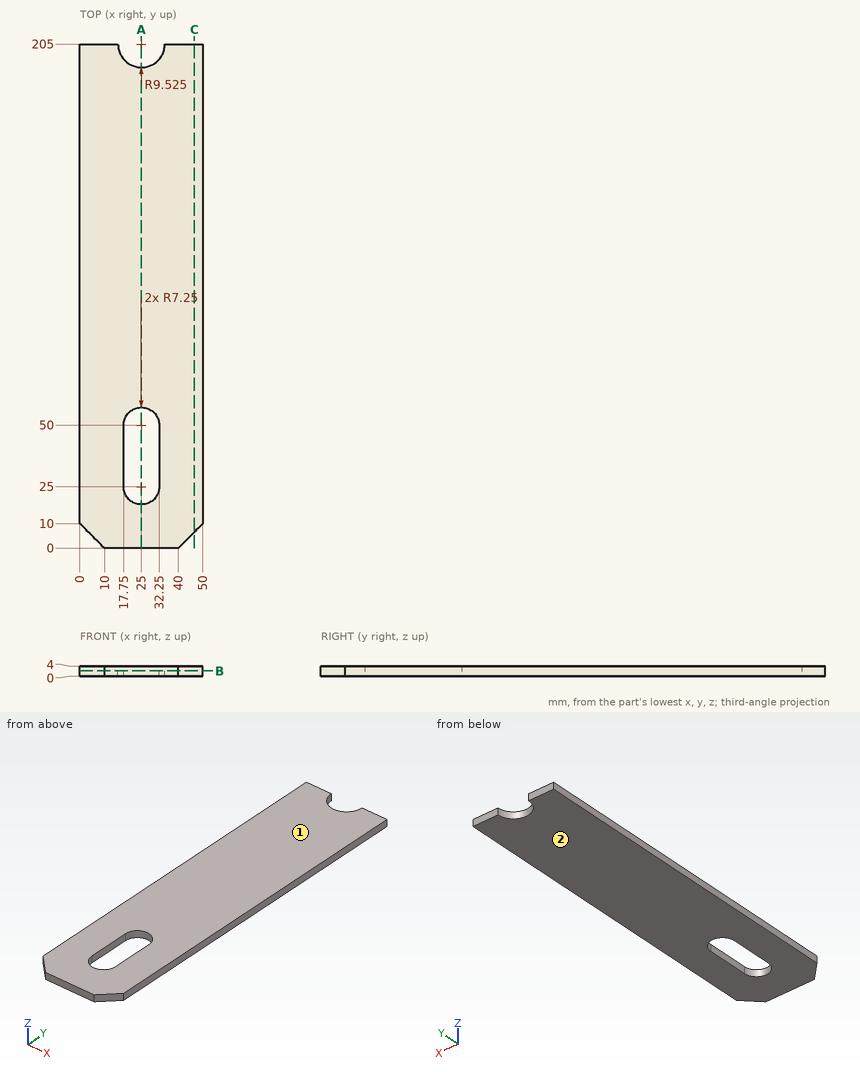
Verification items for this drawing (mm, ordinates from the low corner). Give positions to 0.01 mm unless a question says otherwise; leave off trailing zeros. Loops run counter-clockwise (first coordinate to the right, second up) from the corner with the lowest first, then second, coordinate; pieces in that order, holes last. Notation, with made-up numbers: M 8,72.5 L 15,72.5 A25 ccw 15,93.5 Z; hole C -10.5,8.25 d4. An arc over 180 degrees is marked long. Answer as a JSON object with one key per item and string values. Group by question number.
Item 1: Sectioned sample at B-B on z = 2.1. Record the boundary of the cut face in (x, y) (3 decimals).
Item 2: Material ranges on L1, parallel to X at y = 33.5, z = 0.3; L2, parallel to Y at x = 30.5, z = 3.7; L3, parallel to Y at x = 27, z = 2.4, recorded low to high.
Item 3: Sectioned sample at A-A on x = 25. Record the boundary of the cut face in (y, z) (3 decimals), plus the area to 3 significant figures.
Item 4: Mould release check, pull along Z, two halves, no side actions. Record for the marked faces 1 and 2: pulls with the +Z half, pulls with the -Z half, needs draft (parallel to the pull), parting line crosses it, or undercut.
Item 5: Sectioned sample at C-C on x = 46.5. Record the boundary of the cut face in (y, z).
Findings below:
{
 "1": {"outline": "M 0,10 L 10,0 L 40,0 L 50,10 L 50,205 L 34.525,205 A9.525 cw 15.475,205 L 0,205 Z; hole M 17.75,25 A7.25 ccw 32.25,25 L 32.25,50 A7.25 ccw 17.75,50 Z"},
 "2": {"L1": "0 to 17.75, 32.25 to 50", "L2": "0 to 20.28, 54.72 to 197.22", "L3": "0 to 18.03, 56.97 to 195.69"},
 "3": {"outline": "M 0,0 L 17.75,0 L 17.75,4 L 0,4 Z; M 57.25,0 L 195.475,0 L 195.475,4 L 57.25,4 Z", "area": "624 mm2"},
 "4": {"face 1": "pulls with the +Z half", "face 2": "pulls with the -Z half"},
 "5": {"outline": "M 6.5,0 L 205,0 L 205,4 L 6.5,4 Z"}
}
